The listing builds one solid part. Answer for the finished solid, in the listing's coordinates (mm). Face numbers are marked on the shaded views. A direction names the side the tool comes from. Give positions to 0.01 mm unless a question says otherwise; leave off trailing zeros. Write each loop counter-clockwise with the first axis right and the second up, starting at its lowest first coordinate (ties: lowest second). Pieces come first, ordered by that corner, then holes. Notation, with made-up numbers: (16, -19) -> (37, -19) arc R12 ccw to (37, -9) -> close; hole circle Ø6 at (60, 52). An arc over 180 degrees is marked (long way). Put each result on its own line as item: value. Start each with the question number.
1) A cutting plane is placed at C-C (z = 8). Write down the section's boundary in (x, y), then the cut area to 3 significant figures.
2) A cutting plane is placed at D-D (x = 24). Write down the section's boundary in (y, z), then the cut area to 3 significant figures.
3) For a pull along X with two mould halves and no side action, classify the marked faces 1, 2 and 3 as released by +X, released by -X, zero draft, split by the parting line, or undercut.
4) Find the intervals of material crossed by line 1 along X through (y, z) = (-46.5, -0.5); line 2 along Z through (x, y) = (0, -27.5); line 3 along Z through (x, y) = (83.5, -36), in increasing order. Write a range as from..to.
5) A cutting plane is placed at B-B (x = 0). Write down the section's boundary in (y, z).
6) For the marked faces 4, 5, 6 and 7, determine the directions among +Z, -Z, +X, -X, +Y, -Y from which every point of the face is accessible in a straight line to the end or side of a thin tool.
7) Flat-ended cylindrical pins translate along their axes: pin 1 Ø5 at (x, y) = (22, -44) entering from -Z; pin 2 Ø12.5 at (y, z) = (-36, -23.5) entering from +X; pin 3 Ø3 at (y, z) = (-14, -11.5) entering from +X. Find the tip coordinate at first contact, or state that the pin passes through.
8) A cutting plane is placed at A-A (y = -7). Write down the section's boundary in (x, z), then the cut area to 3 significant figures.
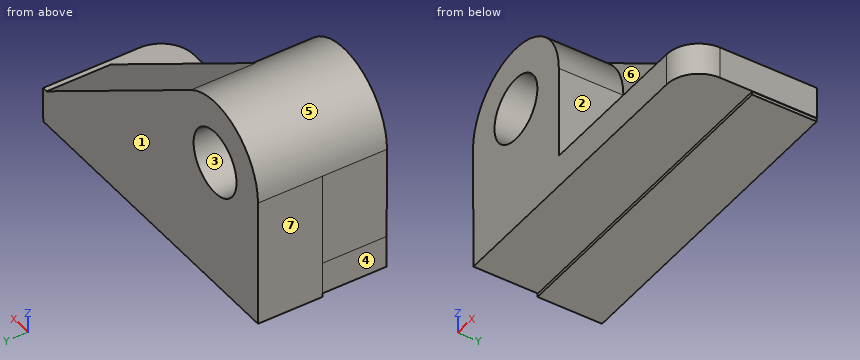
from build123d import *

# Parameters (mm, degrees)
F0_R     = 12.7
F1_DEPTH = 25.4
F2_R     = 12.7
F3_DEPTH = 50.8
F4_R     = 12.7


with BuildPart() as f1:
    # F0 (on Front) → F1 (new body)
    with BuildSketch(Plane.XZ):
        with BuildLine():
            Line((101.6, -38.1), (14.237873, 21.034328))
            ThreePointArc((14.237873, 21.034328), (-11.906259, 22.436599), (-25.4, 0))
            Line((-25.4, 0), (-25.4, -50.8))
            Line((-25.4, -50.8), (101.6, -50.8))
            Line((101.6, -50.8), (101.6, -38.1))
        make_face()
        Circle(F0_R, mode=Mode.SUBTRACT)
    extrude(amount=F1_DEPTH)

    # F2 (on Front) → F3 (join)
    with BuildSketch(Plane.XZ):
        with BuildLine():
            Line((25.4, -36.83), (25.4, 0))
            ThreePointArc((25.4, 0), (0, 25.4), (-25.4, 0))
            Line((-25.4, 0), (-25.183568, -36.83))
            Line((-25.183568, -36.83), (-25.183568, -49.53))
            Line((-25.183568, -49.53), (101.816432, -49.53))
            Line((101.816432, -49.53), (101.816432, -36.83))
            Line((101.816432, -36.83), (25.4, -36.83))
        make_face()
        Circle(F2_R, mode=Mode.SUBTRACT)
    extrude(amount=F3_DEPTH)

    # F4
    f4_edges = [f1.edges().sort_by_distance(p)[0] for p in [
        (101.816432, -50.8, -43.18),
    ]]
    fillet(f4_edges, radius=F4_R)


solid = f1.part
Reply:
1. outline: (-24.11, -50.8) -> (-9.86, -50.8) -> (-9.86, 0) -> (-24.11, 0) -> close; (9.86, -50.8) -> (24.11, -50.8) -> (24.11, -25.4) -> (33.49, -25.4) -> (33.49, 0) -> (9.86, 0) -> close
1. area: 1,690 mm2
2. outline: (-50.8, -49.53) -> (-25.4, -49.53) -> (-25.4, -50.8) -> (0, -50.8) -> (0, 14.43) -> (-25.4, 14.43) -> (-25.4, 8.32) -> (-50.8, 8.32) -> close
2. area: 3,130 mm2
3. face 1: zero draft
3. face 2: released by +X
3. face 3: undercut
4. line 1: x = -25.4..-12.69, 12.69..25.4
4. line 2: z = -49.53..-12.7, 12.7..25.4
4. line 3: z = -49.53..-36.83
5. outline: (-50.8, -49.53) -> (-25.4, -49.53) -> (-25.4, -50.8) -> (0, -50.8) -> (0, -12.7) -> (-50.8, -12.7) -> close; (-50.8, 12.7) -> (0, 12.7) -> (0, 25.4) -> (-50.8, 25.4) -> close
6. face 4: -Z, -X, -Y
6. face 5: +Z, -Y
6. face 6: +Z, +X, -Y
6. face 7: +Z, -Z, -X, +Y, -Y
7. pin 1: stops at z = -49.53
7. pin 2: stops at x = 25.4
7. pin 3: stops at x = 64.52
8. outline: (-25.4, -50.8) -> (101.6, -50.8) -> (101.6, -49.53) -> (101.82, -49.53) -> (101.82, -36.83) -> (99.72, -36.83) -> (14.24, 21.03) arc R25.4 ccw to (-25.4, 0) -> close; hole circle Ø25.4 at (0, 0)
8. area: 6,050 mm2
